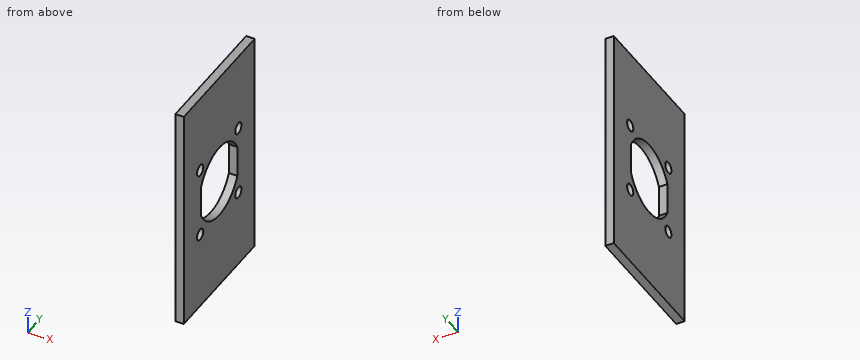
Autodesk Inventor part; units mm, degrees
ref_plane "YZ Plane" through (0, 0, 0) normal (1, 0, 0) x (0, 1, 0)
ref_plane "XZ Plane" through (0, 0, 0) normal (0, 1, 0) x (-1, 0, 0)
ref_plane "XY Plane" through (0, 0, 0) normal (0, 0, 1) x (1, 0, 0)
sketch "スケッチ1" plane through (0, 0, 0) normal (1, 0, 0) x (0, 1, 0)
  line L0 (0, 0) -> (46, 0)
  line L1 (46, 0) -> (46, -80)
  line L2 (46, -80) -> (0, -80)
  line L3 (0, -80) -> (0, 0)
  dimension "d0" = 46
  dimension "d1" = 80
extrude "押し出し1" add sketch "スケッチ1" along normal blind 3
sketch "スケッチ2" plane through (3, 0, 0) normal (1, 0, 0) x (0, 0, -1)
  circle A0 centre (40, 23) radius 13
  line L0 (34.4379, 34.75) -> (45.5621, 34.75)
  line L1 (34.4379, 11.25) -> (45.5621, 11.25)
  line L2 (80, 46) -> (0, 46)
  line L3 (0, 46) -> (0, 0)
  dimension "d4" = 26
  dimension "d7" = 23
  dimension "d8" = 40
  dimension "d9" = 23.5
extrude "押し出し2" cut sketch "スケッチ2" against normal blind 3 contours A0 L1 L0
sketch "スケッチ3" plane through (3, 0, 0) normal (1, 0, 0) x (0, 0, -1)
  circle A0 centre (40, 23) radius 17.5 construction
  arc A1 (34.4379, 34.75) -> (34.4379, 11.25) centre (40, 23) ccw
  arc A2 (45.5621, 11.25) -> (45.5621, 34.75) centre (40, 23) ccw
  line L0 (22.5, 23) -> (57.5, 23) construction
  line L1 (40, 5.5) -> (40, 40.5) construction
  line L2 (40, 23) -> (52.3744, 35.3744) construction
  line L3 (40, 23) -> (57.5, 23) construction
  line L4 (52.3744, 35.3744) -> (27.6256, 10.6256) construction
  line L5 (40, 23) -> (52.3744, 10.6256) construction
  line L6 (27.6256, 35.3744) -> (40, 23) construction
  circle A3 centre (52.3744, 35.3744) radius 2.15
  circle A4 centre (52.3744, 10.6256) radius 2.15
  circle A5 centre (27.6256, 10.6256) radius 2.15
  circle A6 centre (27.6256, 35.3744) radius 2.15
  point P0 (0, 0)
  dimension "d12" = 35
  dimension "d13" = 45
  dimension "d14" = 4.3
  dimension "d15" = 4.3
  dimension "d16" = 4.3
  dimension "d17" = 4.3
hole "穴1" at (3, 35.3744, -27.6256) at (3, 35.3744, -52.3744) at (3, 10.6256, -52.3744) at (3, 10.6256, -27.6256) direction (-1, 0, 0) diameter 4 depth 3
equation "\"BendRadius\" = Thickness"
equation "\"BendReliefWidth\" = Thickness"
equation "\"BendReliefDepth\" = 0.5 * Thickness"
equation "\"CornerReliefSize\" = 4 * Thickness"
equation "\"MinimumRemnant\" = 2 * Thickness"
equation "\"TransitionRadius\" = BendRadius"
equation "\"JacobiRadiusSize\" = BendRadius"
equation "\"GapSize\" = Thickness"
properties part number "nhk28"
Check sheet for the modelled part. Datum: model origin and axes. Units: mm. Round coordinates to 2 decimals unless told otherwise and drop trailing zeros. Loops run counter-clockwise (first coordinate to the right, second up) from the corner with the lowest first, then second, coordinate; pieces in that order, holes last. Notation, with made-up numbers: (2, 58) -> (57, 58) arc R18 cw to (57, 86) -> close; hole circle Ø6 at (-10.75, 60.25). An arc over 180 degrees is marked (long way). Put each result on its own line as item: value. Start each with the question number.
1. Section check A-A (y = 20). Enter the section's corners in (x, z).
2. Section check B-B (z = -28.5). Enter the section's corners in (x, y).
3. Gauge pin test, flat end, axial feed: pin 1 (3.5 mm diameter, centred on y = 35.37, z = -27.63, fed in from +X). Record the tip position at first contact, or that the pin passes through.
4. Section check C-C (x = 2.2). Enter the section's corners in (y, z), plus the area to 3 significant figures.
5. Scan lines: probe 1 along Y at (x, z) = (1.05, -42); probe 2 along Z at (x, y) = (1.1, 36.5); probe 3 along Z at (x, y) = (2, 20.5). Record each from-to range of solid material in increasing order.
6. Section check D-D (y = 30). Enter the section's corners in (x, z), plus the area to 3 significant figures.
Findings:
1. outline: (0, -80) -> (3, -80) -> (3, -52.65) -> (0, -52.65) -> close; (0, -27.35) -> (3, -27.35) -> (3, 0) -> (0, 0) -> close
2. outline: (0, 0) -> (3, 0) -> (3, 8.83) -> (0, 8.83) -> close; (0, 12.42) -> (3, 12.42) -> (3, 16.94) -> (0, 16.94) -> close; (0, 29.06) -> (3, 29.06) -> (3, 33.58) -> (0, 33.58) -> close; (0, 37.17) -> (3, 37.17) -> (3, 46) -> (0, 46) -> close
3. pin 1: passes through
4. outline: (0, -80) -> (46, -80) -> (46, 0) -> (0, 0) -> close; hole circle Ø4 at (10.63, -52.37); hole circle Ø4 at (10.63, -27.63); hole (11.25, -45.56) arc R13 ccw to (34.75, -45.56) -> (34.75, -34.44) arc R13 ccw to (11.25, -34.44) -> close; hole circle Ø4 at (35.37, -52.37); hole circle Ø4 at (35.37, -27.63)
4. area: 3,120 mm^2
5. probe 1: y = 0 to 11.25, 34.75 to 46
5. probe 2: z = -80 to -54.03, -50.72 to -29.28, -25.97 to 0
5. probe 3: z = -80 to -52.76, -27.24 to 0
6. outline: (0, -80) -> (3, -80) -> (3, -50.95) -> (0, -50.95) -> close; (0, -29.05) -> (3, -29.05) -> (3, 0) -> (0, 0) -> close
6. area: 174 mm^2
